The drawing under review shows one solid part. Ordinate dimensions are in mm from its lowest x, y, z. Coordinates: 2 decimals unless noted, no trailing zeros. Order: outer loops, then holes, each group sorted by start corner. A loop starts at its lowest first (then second) coordinate and runs counter-clockwise, first axis right, second up. Notation, with made-up numbers: (-3, 66.5) -> (56, 66.5) arc R23 cw to (56, 92.5) -> close; hole circle Ø8 at (72, -22.5). An arc over 180 degrees is marked (long way). Use a Markdown table: item, result. Add a question column.
Q1. Insertion check: pin 1 (1 mm diameter, centred on x = 2, z = 19.5, fed in from +Y); pin 2 (0.5 mm diameter, centred on x = 2, y = 3, fed in from -Z); pin 3 (1.1 mm diameter, centred on x = 1.5, z = 3, fed in from +Y). Each pin has a flat end and moves straight along its axis. Give the tip position at first contact, or say it passes through.
Q2. Add section A-A (x = 1.5). State the section outline as (y, z) points.
Q3. Wall thickness on probe 1 along Z at (x, y) = (2.15, 2.8); probe 2 along Y at (x, z) = (1.45, 18); probe 3 along X at (y, z) = (1.1, 35): over which ranges is each line inside the solid? List them lowest first.
Q4. Add section C-C (y = 0.7). State the section outline as (x, z) points.
Q5. Add section B-B (z = 17.5). State the section outline as (x, y) points, then the cut area to 3 significant figures.
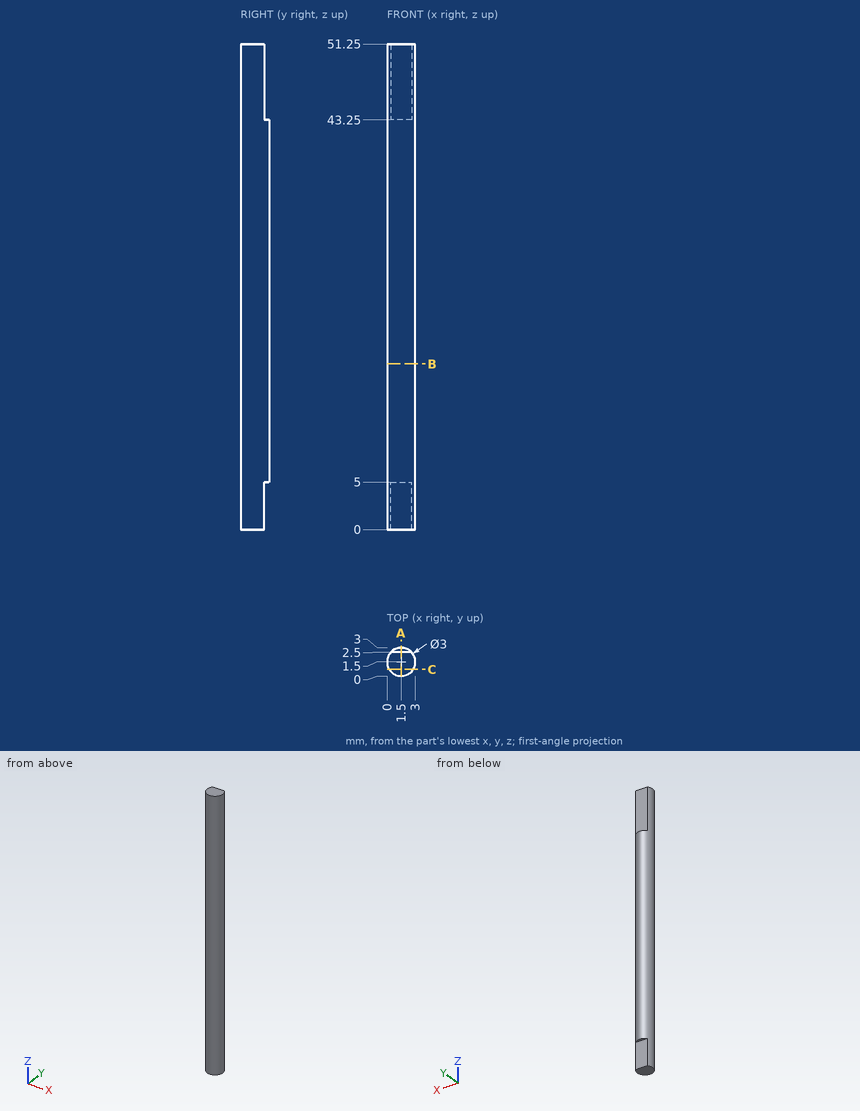
Established:
| question | item | result |
|---|---|---|
| 1 | pin 1 | y = 3 |
| 1 | pin 2 | z = 5 |
| 1 | pin 3 | y = 2.5 |
| 2 | outline | (0, 0) -> (2.5, 0) -> (2.5, 5) -> (3, 5) -> (3, 43.25) -> (2.5, 43.25) -> (2.5, 51.25) -> (0, 51.25) -> close |
| 3 | probe 1 | 5 to 43.25 |
| 3 | probe 2 | 0 to 3 |
| 3 | probe 3 | 0.05 to 2.95 |
| 4 | outline | (0.23, 0) -> (2.77, 0) -> (2.77, 51.25) -> (0.23, 51.25) -> close |
| 5 | outline | circle Ø3 at (1.5, 1.5) |
| 5 | area | 7.07 mm^2 |
